Geometry check sheet. Reference: the model listing, model coordinates, mm. A direction names the side the tool comes from. Round coordinates to 2 decimals unless told otherwise and drop trailing zeros. Write each loop counter-clockwise with the first axis right and the second up, starting at its lowest first coordinate (ties: lowest second). Pieces come first, ordered by that corner, then holes. Notation, with made-up numbers: (77.5, 19.5) - (94.5, 19.5) arc R21 cw to (94.5, 54.5) - close; hole circle Ø9 at (53.25, 49.25). An arc over 180 degrees is marked (long way). Return JSON: item names as keys, results as strings.
Autodesk Inventor part; units mm, degrees
ref_plane "YZ Plane" through (0, 0, 0) normal (1, 0, 0) x (0, 1, 0)
ref_plane "XZ Plane" through (0, 0, 0) normal (0, 1, 0) x (-1, 0, 0)
ref_plane "XY Plane" through (0, 0, 0) normal (0, 0, 1) x (1, 0, 0)
sketch "Sketch1" plane through (0, 0, 0) normal (0, 0, 1) x (1, 0, 0)
  circle A0 centre (0, 0) radius 7.5
  line L0 (-16, 7.5) -> (16, 7.5)
  line L1 (16, 7.5) -> (16, -9.5)
  line L2 (16, -9.5) -> (-16, -9.5)
  line L3 (-16, -9.5) -> (-16, 7.5)
  line L4 (-7.5, 0) -> (-7.5, 7.5)
  line L5 (7.5, 0) -> (7.5, 7.5)
  point P0 (0, -9.5)
  dimension "d0" = 15
  dimension "d5" = 32
  dimension "d6" = 2
extrude "Extrusion1" add sketch "Sketch1" along normal blind 24.2 contours A0 L5 L0 L1 L2 L3 L4
sketch "Sketch2" plane through (0, 0, 24.2) normal (0, 0, 1) x (1, 0, 0)
  line L0 (-16, -9.5) -> (16, -9.5)
  line L1 (16, -9.5) -> (16, 7.5)
  line L2 (16, 7.5) -> (7.5, 7.5)
  line L3 (7.5, 7.5) -> (7.5, 0)
  arc A0 (-7.5, 0) -> (7.5, 0) centre (0, 0) ccw
  line L4 (-7.5, 0) -> (-7.5, 7.5)
  line L5 (-7.5, 7.5) -> (-16, 7.5)
  line L6 (-16, 7.5) -> (-16, -9.5)
  circle A1 centre (0, 0) radius 4.25
  line L7 (-7.5, 7.5) -> (-16, 7.5)
  line L8 (-7.5, 7.5) -> (7.5, 7.5)
  dimension "d10" = 8.5
extrude "Extrusion3" add sketch "Sketch2" along normal blind 3
sketch "Sketch4" plane through (0, 0, 0) normal (0, 0, -1) x (-1, 0, 0)
  line L0 (-16, 7.5) -> (-7.5, 7.5)
  line L1 (-16, -9.5) -> (-16, 7.5)
  line L2 (16, -9.5) -> (-16, -9.5)
  line L3 (16, 7.5) -> (16, -9.5)
  line L4 (7.5, 7.5) -> (16, 7.5)
  line L5 (-7.5, 7.5) -> (7.5, 7.5)
  circle A0 centre (0, 0) radius 4.25
extrude "Extrusion4" add sketch "Sketch4" along normal blind 3
sketch "Sketch5" plane through (0, 0, -3) normal (0, 0, -1) x (-1, 0, 0)
  line L0 (16, 7.5) -> (-16, 7.5)
  line L1 (16, -9.5) -> (16, 7.5)
  line L2 (-16, -9.5) -> (16, -9.5)
  line L3 (-16, 7.5) -> (-16, -9.5)
  circle A0 centre (0, 0) radius 7.5
  arc A1 (-7.5, 0) -> (7.5, 0) centre (0, 0) ccw
  line L4 (7.5, 0) -> (7.5, 7.5)
  line L5 (-16, 7.5) -> (16, 7.5)
  line L6 (-7.5, 7.5) -> (-7.5, 0)
  line L7 (-7.5, 0) -> (-7.5, 7.5)
extrude "Extrusion5" add sketch "Sketch5" along normal blind 130 contours L1 L2 L3 L0 L6 A0 L4
sketch "Sketch6" plane through (0, 0, -133) normal (0, 0, -1) x (-1, 0, 0)
  line L0 (0, 0) -> (0, -9.5) construction
  line L1 (16, -9.5) -> (-16, -9.5) construction
  line L2 (-16, 7.5) -> (-16, -9.5) construction
  point P0 (-12.5, -6)
  point P1 (12.5, -6)
  dimension "d17" = 3.5
  dimension "d18" = 3.5
hole "Hole1" at (12.5, -6, -133) at (-12.5, -6, -133) direction (0, 0, 1) diameter 2.3813 depth 10 tip angle 118
sketch "Sketch7" plane through (-16, 7.5, 27.2) normal (0, 1, 0) x (1, 0, 0)
  line L0 (16, 0) -> (16, 160.2) construction
  line L1 (32, 160.2) -> (0, 160.2)
  line L2 (0, 160.2) -> (0, 0)
  line L3 (32, 0) -> (0, 0)
  point P0 (16, 27.2)
  point P1 (3.5, 3.5)
  point P2 (3.5, 33.5)
  point P3 (3.5, 63.5)
  point P4 (3.5, 93.5)
  point P5 (3.5, 123.5)
  point P6 (3.5, 145.2)
  point P7 (28.5, 3.5)
  point P8 (28.5, 33.5)
  point P9 (28.5, 63.5)
  point P10 (28.5, 93.5)
  point P11 (28.5, 123.5)
  point P12 (28.5, 145.2)
  dimension "d27" = 3.5
  dimension "d44" = 30
  dimension "d49" = 3.5
  dimension "d50" = 15
hole "Hole3" at (-12.5, 7.5, 23.7) at (-12.5, 7.5, -6.3) at (-12.5, 7.5, -36.3) at (-12.5, 7.5, -66.3) at (-12.5, 7.5, -96.3) at (-12.5, 7.5, -118) at (12.5, 7.5, 23.7) at (12.5, 7.5, -6.3) at (12.5, 7.5, -36.3) at (12.5, 7.5, -66.3) at (12.5, 7.5, -96.3) at (12.5, 7.5, -118) direction (0, -1, 0) diameter 2.3813 depth 10 tip angle 118
properties part number "body_v2"
(1) Gauge pin test, flat ends, axial feed: pin 1 (1.5 mm diameter, centred on x = -2, z = -38, fed in from +Y); pin 2 (1.9 mm diameter, centred on x = -12.5, z = -36.3, fed in from +Y). Record the tip position at first contact, or that the pin passes through.
Response values:
{"pin 1": "stops at y = -6.98", "pin 2": "stops at y = -2.64"}
(2) Material ranges on line 1 along X through (y, z) = (1, 23.7); line 2 along X through (y, z) = (1.75, -33); line 3 along Z through (x, y) = (5, -0.5), recorded low to high. Write a range as [from, to].
Response values:
{"line 1": "x = [-16, -13.69], [-11.31, -7.5], [7.5, 11.31], [13.69, 16]", "line 2": "x = [-16, -7.5], [7.5, 16]", "line 3": "z = [-3, 0], [24.2, 27.2]"}
(3) Section check B-B, the plane x = -2. Enter the section's corners in (y, z), plus the area to 3 significant figures.
Response values:
{"outline": "(-9.5, -133) - (-7.23, -133) - (-7.23, -3) - (-3.75, -3) - (-3.75, 0) - (-7.23, 0) - (-7.23, 24.2) - (-3.75, 24.2) - (-3.75, 27.2) - (-9.5, 27.2) - close; (3.75, -3) - (7.5, -3) - (7.5, 0) - (3.75, 0) - close; (3.75, 24.2) - (7.5, 24.2) - (7.5, 27.2) - (3.75, 27.2) - close", "area": "407 mm^2"}
(4) Access from +Z, -Z, +X, -X, +Y, -Y to the whole of each face (thin tool, end or side, straight path). Record for faces 4 (the face through (-0.16, -7.5, -67.09)), 5 (the face through (-7.5, 4, 12)), 6 (the face through (-2.285, -3.584, -1.479)).
Response values:
{"face 4": "-Z, +Y", "face 5": "+Y", "face 6": "+Z, -Z"}
(5) Release check for a two-part mould opening along Z. For faces 1 (the face through (-16, -1, -52)), 2 (the face through (0.16, -7.5, 11.93)), 3 (the face through (-3.2, 3.4, -3)) record: pulls with the +Z half, pulls with the -Z half, needs draft (parallel to the pull), parting line crosses it, or undercut.
Response values:
{"face 1": "needs draft", "face 2": "undercut", "face 3": "pulls with the -Z half"}
(6) Section check C-C, the plane x = 6. Enter the section's corners in (y, z).
Response values:
{"outline": "(-9.5, -133) - (-4.5, -133) - (-4.5, -3) - (7.5, -3) - (7.5, 0) - (-4.5, 0) - (-4.5, 24.2) - (7.5, 24.2) - (7.5, 27.2) - (-9.5, 27.2) - close"}
(7) Section check A-A, the plane y = 2.5. Give the number of separate pieces and of enclosed holes in the cut face, plus the area to 3 significant figures.
Response values:
{"separate pieces": "2", "enclosed holes": "12", "area": "2,720 mm^2"}
